Part model, mm, in its own coordinate system. Face numbers are marked on the shaded views. Give positions to 0.01 mm unless a question says otherwise; leave off trailing zeros. Write each loop counter-clockwise with the first axis right and the second up, starting at its lowest first coordinate (ties: lowest second). Pieces come first, ordered by that corner, then holes. Notation, with made-up numbers: M -35,10.25 L -6,10.25 A35 cw -6,49.25 Z; hole C 53,29 d10. An arc over 180 degrees is marked long. Use a Markdown table: item, result.
```python
from build123d import *

# Parameters (mm, degrees)
F0_R     = 130
F0_R_2   = 5.25
F0_R_3   = 103.9
F1_DEPTH = 15
F0_R_4   = 95
F0_R_5   = 45
F2_DEPTH = 42


with BuildPart() as f1:
    # F0 (on Front) → F1 (new body)
    with BuildSketch(Plane.XZ):
        Circle(F0_R)
        with Locations((-54.3090440333, -105.6210622191)):
            Circle(F0_R_2, mode=Mode.SUBTRACT)
        with Locations((54.3090440333, -105.6210622191)):
            Circle(F0_R_2, mode=Mode.SUBTRACT)
        with Locations((-119.4707155228, 0)):
            Circle(F0_R_2, mode=Mode.SUBTRACT)
        with Locations((-54.3090440333, 105.6210622191)):
            Circle(F0_R_2, mode=Mode.SUBTRACT)
        Circle(F0_R_3, mode=Mode.SUBTRACT)
        with Locations((119.4707155228, 0)):
            Circle(F0_R_2, mode=Mode.SUBTRACT)
        with Locations((54.3090440333, 105.6210622191)):
            Circle(F0_R_2, mode=Mode.SUBTRACT)
    extrude(amount=F1_DEPTH)

    # F0 (on Front) → F2 (join)
    with BuildSketch(Plane.XZ):
        Circle(F0_R_3)
        Circle(F0_R_4, mode=Mode.SUBTRACT)
        Circle(F0_R_4)
        with BuildLine():
            ThreePointArc((69.6607525504, 60.094754797), (85.33124775, 34.3886341314), (91.8640299573, 5))
            ThreePointArc((91.8640299573, 5), (91.9660012072, 2.5009242218), (92, 0))
            ThreePointArc((92, 0), (91.9660012072, -2.5009242218), (91.8640299573, -5))
            ThreePointArc((91.8640299573, -5), (85.33124775, -34.3886341314), (69.6607525504, -60.094754797))
            ThreePointArc((69.6607525504, -60.094754797), (66.2917791865, -63.7918491054), (62.7268559085, -67.3003829694))
            ThreePointArc((62.7268559085, -67.3003829694), (36.0218675411, -84.6547403212), (5, -91.8640299573))
            ThreePointArc((5, -91.8640299573), (0, -92), (-5, -91.8640299573))
            ThreePointArc((-5, -91.8640299573), (-36.0218675411, -84.6547403212), (-62.7268559085, -67.3003829694))
            ThreePointArc((-62.7268559085, -67.3003829694), (-66.2917791865, -63.7918491054), (-69.6607525504, -60.094754797))
            ThreePointArc((-69.6607525504, -60.094754797), (-85.33124775, -34.3886341314), (-91.8640299573, -5))
            ThreePointArc((-91.8640299573, -5), (-92, 0), (-91.8640299573, 5))
            ThreePointArc((-91.8640299573, 5), (-85.33124775, 34.3886341314), (-69.6607525504, 60.094754797))
            ThreePointArc((-69.6607525504, 60.094754797), (-66.2917791865, 63.7918491054), (-62.7268559085, 67.3003829694))
            ThreePointArc((-62.7268559085, 67.3003829694), (-36.0218675411, 84.6547403212), (-5, 91.8640299573))
            ThreePointArc((-5, 91.8640299573), (0, 92), (5, 91.8640299573))
            ThreePointArc((5, 91.8640299573), (36.0218675411, 84.6547403212), (62.7268559085, 67.3003829694))
            ThreePointArc((62.7268559085, 67.3003829694), (66.2917791865, 63.7918491054), (69.6607525504, 60.094754797))
        make_face(mode=Mode.SUBTRACT)
        with BuildLine():
            ThreePointArc((49.7493718553, -5), (49.9373036555, -2.503138753), (50, 0))
            ThreePointArc((50, 0), (49.9373036555, 2.503138753), (49.7493718553, 5))
            ThreePointArc((49.7493718553, 5), (46.375678125, 18.6894750714), (39.3144958612, 30.8928861582))
            ThreePointArc((39.3144958612, 30.8928861582), (36.0281408622, 34.6694832095), (32.3805992193, 38.0985143306))
            ThreePointArc((32.3805992193, 38.0985143306), (19.5771019245, 46.0080110441), (5, 49.7493718553))
            ThreePointArc((5, 49.7493718553), (0, 50), (-5, 49.7493718553))
            ThreePointArc((-5, 49.7493718553), (-19.5771019245, 46.0080110441), (-32.3805992193, 38.0985143306))
            ThreePointArc((-32.3805992193, 38.0985143306), (-36.0281408622, 34.6694832095), (-39.3144958612, 30.8928861582))
            ThreePointArc((-39.3144958612, 30.8928861582), (-46.375678125, 18.6894750714), (-49.7493718553, 5))
            ThreePointArc((-49.7493718553, 5), (-50, 0), (-49.7493718553, -5))
            ThreePointArc((-49.7493718553, -5), (-46.375678125, -18.6894750714), (-39.3144958612, -30.8928861582))
            ThreePointArc((-39.3144958612, -30.8928861582), (-36.0281408622, -34.6694832095), (-32.3805992193, -38.0985143306))
            ThreePointArc((-32.3805992193, -38.0985143306), (-19.5771019245, -46.0080110441), (-5, -49.7493718553))
            ThreePointArc((-5, -49.7493718553), (0, -50), (5, -49.7493718553))
            ThreePointArc((5, -49.7493718553), (19.5771019245, -46.0080110441), (32.3805992193, -38.0985143306))
            ThreePointArc((32.3805992193, -38.0985143306), (36.0281408622, -34.6694832095), (39.3144958612, -30.8928861582))
            ThreePointArc((39.3144958612, -30.8928861582), (46.375678125, -18.6894750714), (49.7493718553, -5))
        make_face()
        Circle(F0_R_5, mode=Mode.SUBTRACT)
        with BuildLine():
            ThreePointArc((5, 49.7493718553), (19.5771019245, 46.0080110441), (32.3805992193, 38.0985143306))
            Line((32.3805992193, 38.0985143306), (62.7268559085, 67.3003829694))
            ThreePointArc((62.7268559085, 67.3003829694), (36.0218675411, 84.6547403212), (5, 91.8640299573))
            Line((5, 91.8640299573), (5, 49.7493718553))
        make_face()
        with BuildLine():
            ThreePointArc((-32.3805992193, 38.0985143306), (-19.5771019245, 46.0080110441), (-5, 49.7493718553))
            Line((-5, 49.7493718553), (-5, 91.8640299573))
            ThreePointArc((-5, 91.8640299573), (-36.0218675411, 84.6547403212), (-62.7268559085, 67.3003829694))
            Line((-62.7268559085, 67.3003829694), (-32.3805992193, 38.0985143306))
        make_face()
        with BuildLine():
            Line((-5, -91.8640299573), (-5, -49.7493718553))
            ThreePointArc((-5, -49.7493718553), (-19.5771019245, -46.0080110441), (-32.3805992193, -38.0985143306))
            Line((-32.3805992193, -38.0985143306), (-62.7268559085, -67.3003829694))
            ThreePointArc((-62.7268559085, -67.3003829694), (-36.0218675411, -84.6547403212), (-5, -91.8640299573))
        make_face()
        with BuildLine():
            Line((62.7268559085, -67.3003829694), (32.3805992193, -38.0985143306))
            ThreePointArc((32.3805992193, -38.0985143306), (19.5771019245, -46.0080110441), (5, -49.7493718553))
            Line((5, -49.7493718553), (5, -91.8640299573))
            ThreePointArc((5, -91.8640299573), (36.0218675411, -84.6547403212), (62.7268559085, -67.3003829694))
        make_face()
        with BuildLine():
            ThreePointArc((39.3144958612, 30.8928861582), (46.375678125, 18.6894750714), (49.7493718553, 5))
            Line((49.7493718553, 5), (91.8640299573, 5))
            ThreePointArc((91.8640299573, 5), (85.33124775, 34.3886341314), (69.6607525504, 60.094754797))
            Line((69.6607525504, 60.094754797), (39.3144958612, 30.8928861582))
        make_face()
        with BuildLine():
            ThreePointArc((-49.7493718553, 5), (-46.375678125, 18.6894750714), (-39.3144958612, 30.8928861582))
            Line((-39.3144958612, 30.8928861582), (-69.6607525504, 60.094754797))
            ThreePointArc((-69.6607525504, 60.094754797), (-85.33124775, 34.3886341314), (-91.8640299573, 5))
            Line((-91.8640299573, 5), (-49.7493718553, 5))
        make_face()
        with BuildLine():
            Line((-69.6607525504, -60.094754797), (-39.3144958612, -30.8928861582))
            ThreePointArc((-39.3144958612, -30.8928861582), (-46.375678125, -18.6894750714), (-49.7493718553, -5))
            Line((-49.7493718553, -5), (-91.8640299573, -5))
            ThreePointArc((-91.8640299573, -5), (-85.33124775, -34.3886341314), (-69.6607525504, -60.094754797))
        make_face()
        with BuildLine():
            Line((91.8640299573, -5), (49.7493718553, -5))
            ThreePointArc((49.7493718553, -5), (46.375678125, -18.6894750714), (39.3144958612, -30.8928861582))
            Line((39.3144958612, -30.8928861582), (69.6607525504, -60.094754797))
            ThreePointArc((69.6607525504, -60.094754797), (85.33124775, -34.3886341314), (91.8640299573, -5))
        make_face()
    extrude(amount=F2_DEPTH)


solid = f1.part
```
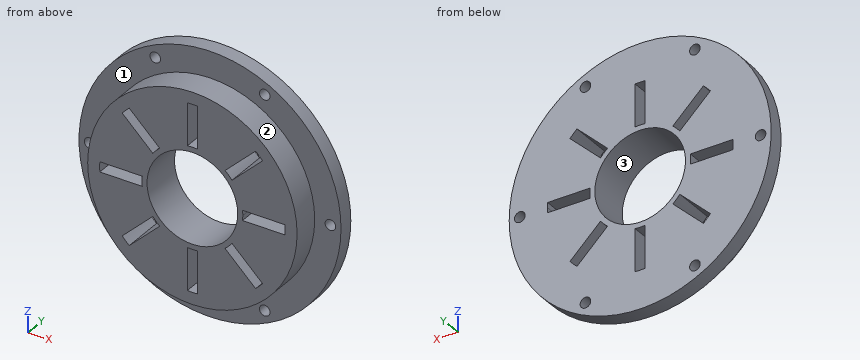
1. Cut at A-A, the plane x = 0. Give the cut face in (y, z).
Findings below:
| item | result |
|---|---|
| outline | M -42,-103.9 L -15,-103.9 L -15,-130 L 0,-130 L 0,-92 L -42,-92 Z; M -42,-50 L 0,-50 L 0,-45 L -42,-45 Z; M -42,45 L 0,45 L 0,50 L -42,50 Z; M -42,92 L 0,92 L 0,130 L -15,130 L -15,103.9 L -42,103.9 Z |
2. Cut at C-C, the plane y = -39. State how many separate pieces and enclosed holes the cut face has, then the cut area to 3 significant figures.
Findings below:
| item | result |
|---|---|
| separate pieces | 1 |
| enclosed holes | 9 |
| area | 24,200 mm2 |
3. Drill centre lines: L1, parallel to X at y = -29, z = 2.5; L2, parallel to Z at x = -33, y = -11.5; L3, parallel to Z at x = 40.5, y = -21. Where is each one in solid material? Low to high.
Findings below:
| item | result |
|---|---|
| L1 | -103.87 to -91.97, -49.94 to -44.93, 44.93 to 49.94, 91.97 to 103.87 |
| L2 | -125.74 to -38.69, -37.56 to -30.59, 30.59 to 37.56, 38.69 to 125.74 |
| L3 | -95.68 to -45.91, -32.03 to -19.62, 19.62 to 32.03, 45.91 to 95.68 |
4. Cut at B-B, the plane z = 26. Give the cut face in (x, y), then the cut area to 3 significant figures.
Findings below:
| item | result |
|---|---|
| outline | M -127.37,-15 L -100.59,-15 L -100.59,-42 L -36.73,-42 L -36.73,0 L -127.37,0 Z; M 36.73,-42 L 100.59,-42 L 100.59,-15 L 127.37,-15 L 127.37,0 L 36.73,0 Z |
| area | 6,170 mm2 |
5. Two-plate mould, pull along Z, no slides. Class the marked faces 1, 2 and 3: released by +Z, released by -Z, zero draft, split by the parting line, or undercut.
Findings below:
| item | result |
|---|---|
| face 1 | zero draft |
| face 2 | split by the parting line |
| face 3 | undercut |
6. Drop flat-ended pins along their axis: P1, Ø8.5, axis at x = 54.31, z = -105.62, coming from the +Y side; P2, Ø13.5, axis at x = 119.47, z = 0, coming from the -Y side; P3, Ø12, axis at x = -61.5, y = -34, coming from the -Z side; P4, Ø1.5, axis at x = -22.5, y = -8, coming from the -Z side. Give the stop position or say it passes through.
Findings below:
| item | result |
|---|---|
| P1 | through |
| P2 | y = -15 |
| P3 | z = -87.83 |
| P4 | z = -128.17 |
